```python
from build123d import *

# Parameters (mm, degrees)
F1_DEPTH = 5.9944
F0_R     = 13.0048
F2_DEPTH = 20.0025
F0_R_2   = 5.9944
F3_DEPTH = 13.0048


with BuildPart() as f1:
    # F0 (on Front) → F1 (new body, symmetric)
    with BuildSketch(Plane.XZ):
        with BuildLine():
            ThreePointArc((-79.938103, 28.535882), (-68.488104, 27.681584), (-62.995777, 17.598595))
            ThreePointArc((-62.995777, 17.598595), (-74.23434, 5.62137), (-86.901777, 16.075807))
            Line((-86.901777, 16.075807), (-86.901777, -22.406405))
            ThreePointArc((-86.901777, -22.406405), (-74.900277, -10.404905), (-62.898777, -22.406405))
            ThreePointArc((-62.898777, -22.406405), (-63.941977, -27.300448), (-66.890221, -31.343686))
            Line((-66.890221, -31.343686), (-4.163324, 24.875419))
            ThreePointArc((-4.163324, 24.875419), (2.722442, 27.884357), (10.046576, 26.203719))
            ThreePointArc((10.046576, 26.203719), (-1.965359, 49.095809), (12.701229, 70.384903))
            Line((12.701229, 70.384903), (-79.938103, 28.535882))
        make_face()
    extrude(amount=F1_DEPTH, both=True)

    # F0 (on Front) → F2 (join, symmetric)
    with BuildSketch(Plane.XZ):
        with BuildLine():
            ThreePointArc((48.002223, 47.595995), (36.558423, 68.604889), (12.701229, 70.384903))
            ThreePointArc((12.701229, 70.384903), (-1.965359, 49.095809), (10.046576, 26.203719))
            ThreePointArc((10.046576, 26.203719), (35.273948, 25.811479), (48.002223, 47.595995))
        make_face()
        with Locations((22.995923, 47.595995)):
            Circle(F0_R, mode=Mode.SUBTRACT)
    extrude(amount=F2_DEPTH, both=True)

    # F0 (on Front) → F3 (join, symmetric)
    with BuildSketch(Plane.XZ):
        with BuildLine():
            ThreePointArc((-86.901777, 16.075807), (-74.23434, 5.62137), (-62.995777, 17.598595))
            ThreePointArc((-62.995777, 17.598595), (-68.488104, 27.681584), (-79.938103, 28.535882))
            ThreePointArc((-79.938103, 28.535882), (-85.473661, 23.453626), (-86.901777, 16.075807))
        make_face()
        with Locations((-74.997277, 17.598595)):
            Circle(F0_R_2, mode=Mode.SUBTRACT)
        with BuildLine():
            ThreePointArc((-62.898777, -22.406405), (-74.900277, -10.404905), (-86.901777, -22.406405))
            ThreePointArc((-86.901777, -22.406405), (-79.79432, -33.364705), (-66.890221, -31.343686))
            ThreePointArc((-66.890221, -31.343686), (-63.941977, -27.300448), (-62.898777, -22.406405))
        make_face()
        with Locations((-74.900277, -22.406405)):
            Circle(F0_R_2, mode=Mode.SUBTRACT)
    extrude(amount=F3_DEPTH, both=True)


solid = f1.part
```
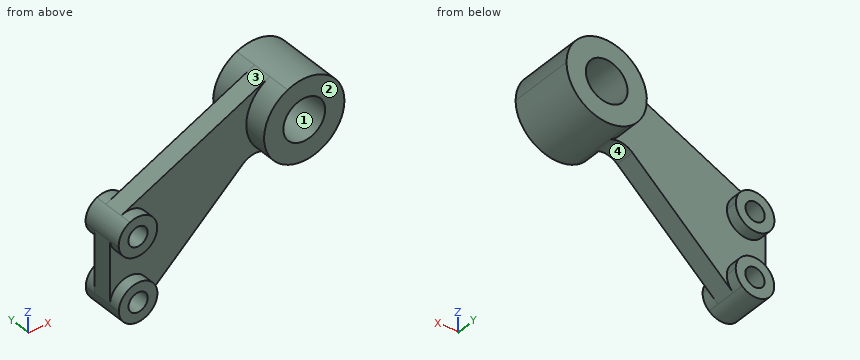
Geometry check sheet. Reference: the model listing, model coordinates, mm. Face numbers are marked on the shaded views. Coordinates: 2 decimals unless noted, no trailing zeros. Order: outer loops, then holes, each group sorted by start corner. A loop starts at its lowest first (then second) coordinate and runs counter-clockwise, first axis right, second up. Notation, with made-up numbers: M 61,-2 L 108,-2 A26 cw 108,26 Z; hole C -29.75,-34.5 d1. An arc over 180 degrees is marked long. One line per question, with ' | ' between items. Start each with the question number.
Item 1: Cross-section at A-A on y = 7.5. Enter the section's corners in (x, z).
Item 2: Cross-section at B-B on x = -73. Enter the section's corners in (y, z), then the cut area to 3 significant figures.
Item 3: Material ranges on L1, parallel to Z at x = -78, y = -7.5; L2, parallel to X at y = 8.5, z = 58.5; L3, parallel to X at y = 11, z = -19.5, recorded low to high. Write a range as [from, to].
Item 4: Cross-section at D-D on x = 33. Enter the section's corners in (y, z).
Item 5: Draft check along Z on the marked faces 1, 2, 3 and 4. Enter one of: pulls with the +Z half, pulls with the -Z half, needs draft (parallel to the pull), parting line crosses it, or undercut.
Item 6: Cross-section at C-C on z = 51.5. Enter the section's corners in (x, y).
Item 7: Gauge pin test, flat ends, axial feed: pin 1 (4 mm diameter, centred on y = -3, z = -4.5, fed in from -X); pin 2 (4 mm diameter, centred on x = -8, z = 24, fed in from +Y); pin 3 (15.5 mm diameter, centred on x = -75, z = 17.6, fed in from -Y). Record the tip position at first contact, or that the pin passes through.
Findings:
1) outline: C -75,17.6 d24; C -74.9,-22.41 d24; M 10.05,26.2 A25.01 ccw 48,47.6 A25.01 ccw long Z; hole C -75,17.6 d11.99; hole C -74.9,-22.41 d11.99; hole C 23,47.6 d26.01
2) outline: M -13,-34.26 L 13,-34.26 L 13,-28.09 L -13,-28.09 Z; M -13,-16.72 L 13,-16.72 L 13,-10.56 L 5.99,-10.56 L 5.99,5.76 L 13,5.76 L 13,11.95 L -13,11.95 L -13,5.76 L -5.99,5.76 L -5.99,-10.56 L -13,-10.56 Z; M -13,23.25 L 13,23.25 L 13,29.43 L 5.99,29.43 L 5.99,31.67 L -5.99,31.67 L -5.99,29.43 L -13,29.43 Z | area: 865 mm²
3) L1: z = [-34, -27.54], [-17.28, -10.81], [5.98, 12.41], [22.79, 29.22] | L2: x = [0.49, 15.91], [30.08, 45.5] | L3: x = [-86.54, -80.14], [-69.66, -63.26]
4) outline: M -20,24.68 L 20,24.68 L 20,39.29 L -20,39.29 Z; M -20,55.91 L 20,55.91 L 20,70.51 L -20,70.51 Z
5) face 1: undercut | face 2: needs draft | face 3: pulls with the +Z half | face 4: pulls with the -Z half
6) outline: M -29.1,-5.99 L -1.7,-5.99 L -1.7,-20 L 10.59,-20 L 10.59,20 L -1.7,20 L -1.7,5.99 L -29.1,5.99 Z; M 35.4,-20 L 47.7,-20 L 47.7,20 L 35.4,20 Z
7) pin 1: stops at x = -86.9 | pin 2: stops at y = 5.99 | pin 3: stops at y = -13
